Answer from the drawing. Dimensions are ordinates in mm from the lowest x, y and z of the part. A direction names the side the tool comes from. Give positions to 0.01 mm unless a question says otherwise; leave off trailing zeros. Loops run counter-clockwise (first coordinate to the right, second up) from the corner with the lowest first, then second, coordinate; pieces in that order, holes last. Notation, with made-up numbers: (25.25, -25) - (71.25, -25) arc R16 cw to (71.25, 2) - close; hole circle Ø6 at (47, -17.5). An arc over 180 degrees is marked (long way). Answer as CSV lines item,"result". Start each with the question number.
1) Flat-ended cylindrical pins translate along their axes: pin 1 (2.5 mm diameter, centred on x = 5.5, z = 5, fed in from +Y); pin 2 (1 mm diameter, centred on x = 48, y = 21, fed in from -Z); pin 3 (1 mm diameter, centred on y = 24, z = 19, fed in from +X); pin 4 (1.5 mm diameter, centred on x = 49, z = 21.5, fed in from +Y). Find the tip coordinate at first contact, or state that the pin passes through.
2) A cutting plane is placed at D-D (x = 80.5). Determine the outline of the cut face in (y, z), and give its area (3 significant figures).
3) A cutting plane is placed at A-A (x = 57). Determine the outline of the cut face in (y, z), and give its area (3 significant figures).
4) A cutting plane is placed at B-B (z = 14.5). Give the number of separate pieces and of enclosed holes in the cut face, and give its area (3 significant figures).
5) A cutting plane is placed at C-C (y = 43). Determine the outline of the cut face in (x, z).
6) Find the intervals of material crossed by line 1 along Y through (x, z) = (45, 2.25); line 2 along Z through (x, y) = (57, 65); line 3 along X through (y, z) = (56, 22), in increasing order.
7) For a pull along X with two mould halves and no side action, classify the marked faces 1, 2 and 3 as pulls with the +X half, pulls with the -X half, needs draft (parallel to the pull), parting line crosses it, or undercut.
8) For the marked faces 4, 5, 6, 7 and 8, determine the directions among +Z, -Z, +X, -X, +Y, -Y from which every point of the face is accessible in a straight line to the end or side of a thin tool.
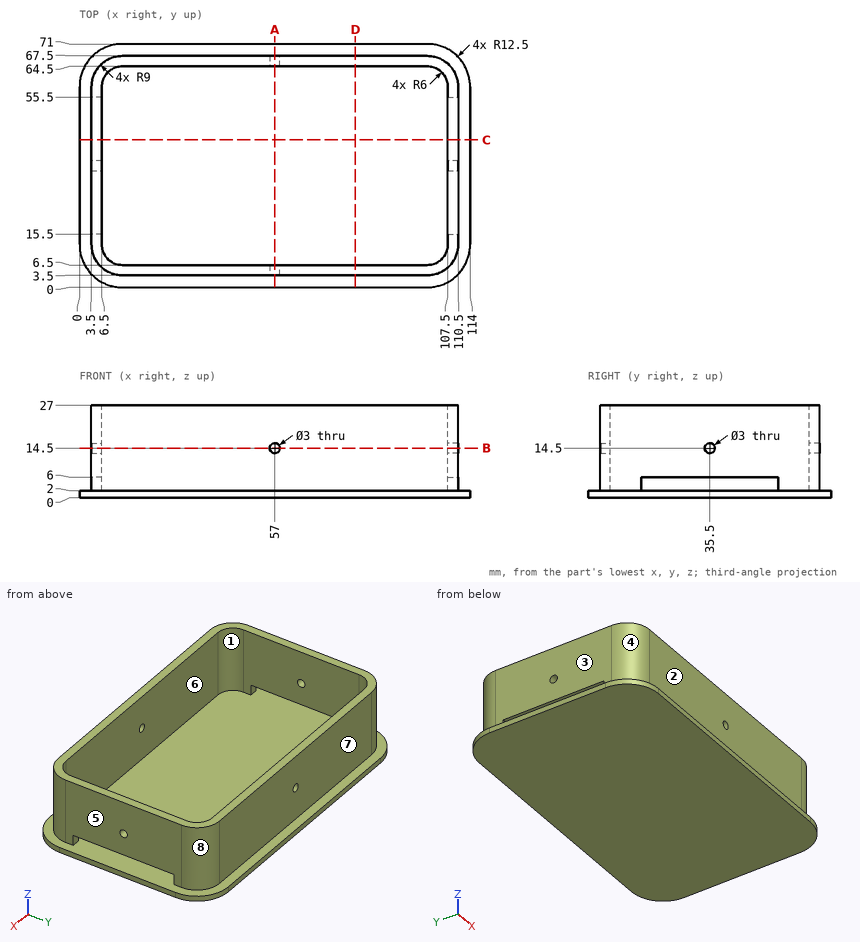
Ans:
1,pin 1,"y = 65.42"
1,pin 2,"z = 0"
1,pin 3,"x = 110.5"
1,pin 4,"y = 67.5"
2,outline,"(0, 0) - (71, 0) - (71, 2) - (67.5, 2) - (67.5, 27) - (64.5, 27) - (64.5, 2) - (6.5, 2) - (6.5, 27) - (3.5, 27) - (3.5, 2) - (0, 2) - close"
2,area,"292 mm2"
3,outline,"(0, 0) - (71, 0) - (71, 2) - (67.5, 2) - (67.5, 13) - (64.5, 13) - (64.5, 2) - (6.5, 2) - (6.5, 13) - (3.5, 13) - (3.5, 2) - (0, 2) - close; (3.5, 16) - (6.5, 16) - (6.5, 27) - (3.5, 27) - close; (64.5, 16) - (67.5, 16) - (67.5, 27) - (64.5, 27) - close"
3,area,"274 mm2"
4,separate pieces,"4"
4,enclosed holes,"0"
4,area,"915 mm2"
5,outline,"(0, 0) - (114, 0) - (114, 2) - (0, 2) - close; (3.5, 6) - (6.5, 6) - (6.5, 27) - (3.5, 27) - close; (107.5, 6) - (110.5, 6) - (110.5, 27) - (107.5, 27) - close"
6,line 1,"3.5 to 6.5, 64.5 to 67.5"
6,line 2,"0 to 13, 16 to 27"
6,line 3,"3.5 to 6.5, 107.5 to 110.5"
7,face 1,"undercut"
7,face 2,"needs draft"
7,face 3,"pulls with the -X half"
8,face 4,"+Z, -X, -Y"
8,face 5,"+Z, +X, +Y, -Y"
8,face 6,"+Z"
8,face 7,"+Z, +X, -X, +Y"
8,face 8,"+Z, +X, +Y"
